Input: part model. Units: mm. Frame: model coordinates. Face numbers are marked on the shaded views. Coordinates: 2 decimals unless noted, no trailing zeros. Write each loop counter-clockwise with the first axis right and the second up, starting at its lowest first coordinate (ties: lowest second). Pieces come first, ordered by that corner, then holes.
1) Pin query (flat end, axial travel): pin 1 Ø1.5 at (x, y) = (4, 12.5) entering from +Z; pin 2 Ø1.6 at (x, y) = (6, 21) entering from -Z (3 decimals); pin 3 Ø0.8 at (x, z) = (-7, 1) entering from +Y; pin 4 Ø0.8 at (y, z) = (9, 0.5) entering from -X. Return the tip coordinate at first contact, or that it passes through.
2) Draft query along X for the marked faces 1, 2 and 3. Return one class per face: pulls with the +X half, pulls with the -X half, needs draft (parallel to the pull), parting line crosses it, or undercut.
3) Section query C-C (y = 16). Output: boundary loops of the cut face in (x, z).
4) Section query A-A (z = 1.9). Output: boundary loops of the cut face in (x, y).
5) Section query B-B (x = 2). Output: boundary loops of the cut face in (y, z).
6) Line query: L1, parallel to Y at x = -6, z = 1.1; L2, parallel to Z at x = -6.5, y = 4.75; L3, parallel to Y at x = 6, z = 2.15. Output: solid intervals per line, ascending.
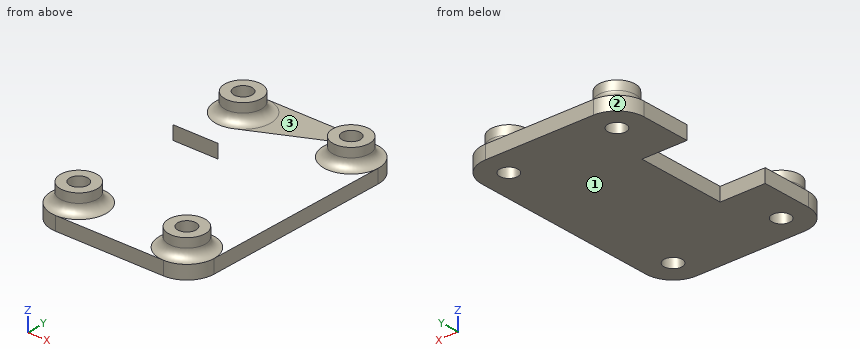
Autodesk Inventor part; units mm, degrees
ref_plane "YZ Plane" through (0, 0, 0) normal (1, 0, 0) x (0, 1, 0)
ref_plane "XZ Plane" through (0, 0, 0) normal (0, 1, 0) x (-1, 0, 0)
ref_plane "XY Plane" through (0, 0, 0) normal (0, 0, 1) x (1, 0, 0)
sketch "Náčrt1" plane through (0, 0, 0) normal (0, 0, 1) x (1, 0, 0)
  circle A0 centre (-6, 0) radius 1
  circle A1 centre (-6, 21) radius 1
  circle A2 centre (6, 0) radius 1
  circle A3 centre (6, 21) radius 1
  arc A4 (-6, 24) -> (-9, 21) centre (-6, 21) ccw
  arc A5 (9, 21) -> (6, 24) centre (6, 21) ccw
  arc A6 (6, -3) -> (9, 0) centre (6, 0) ccw
  arc A7 (-9, 0) -> (-6, -3) centre (-6, 0) ccw
  line L0 (-6, 24) -> (6, 24)
  line L1 (9, 21) -> (9, 0)
  line L2 (-6, -3) -> (6, -3)
  line L3 (-9, 15.5) -> (-4, 15.5)
  line L4 (-9, 5.5) -> (-4, 5.5)
  line L5 (-4, 15.5) -> (-4, 5.5)
  line L6 (-9, 21) -> (-9, 15.5)
  line L7 (-9, 5.5) -> (-9, 0)
  point P0 (0, 0)
  dimension "d0" = 2
  dimension "d2" = 2
  dimension "d4" = 19
  dimension "d5" = 2
  dimension "d6" = 2
  dimension "d7" = 2
  dimension "d8" = 2
  dimension "d9" = 4.5
  dimension "d10" = 5
extrude "Vysunutí1" add sketch "Náčrt1" along normal blind 1.5
sketch "Náčrt3" plane through (0, 0, 1.5) normal (0, 0, 1) x (1, 0, 0)
  circle A0 centre (-6, 21) radius 1
  circle A1 centre (-6, 21) radius 1
  circle A2 centre (6, 21) radius 1
  circle A3 centre (6, 21) radius 1
  circle A4 centre (6, 0) radius 1
  circle A5 centre (6, 0) radius 1
  circle A6 centre (-6, 0) radius 1
  circle A7 centre (-6, 21) radius 2
  circle A8 centre (6, 21) radius 2
  circle A9 centre (6, 0) radius 2
  circle A10 centre (-6, 0) radius 2
  point P0 (0, 0)
  dimension "d13" = 1
  dimension "d14" = 1
  dimension "d15" = 1
  dimension "d16" = 1
extrude "Vysunutí2" add sketch "Náčrt3" along normal blind 2
fillet "Zaoblení1" radius 1 4 edges at (-8, 21, 1.5) (4, 21, 1.5) (-8, 0, 1.5) (4, 0, 1.5)
properties part number "drzak_kamery2"
Answer:
1. pin 1: stops at z = 1.5
1. pin 2: passes through
1. pin 3: stops at y = 23.94
1. pin 4: stops at x = -4
2. face 1: needs draft
2. face 2: pulls with the -X half
2. face 3: undercut
3. outline: (-9, 0) - (9, 0) - (9, 1.5) - (-9, 1.5) - close
4. outline: circle Ø4.4 at (-6, 0); circle Ø4.4 at (-6, 21); circle Ø4.4 at (6, 0); circle Ø4.4 at (6, 21); hole circle Ø2 at (-6, 0); hole circle Ø2 at (-6, 21); hole circle Ø2 at (6, 0); hole circle Ø2 at (6, 21)
5. outline: (-3, 0) - (24, 0) - (24, 1.5) - (-3, 1.5) - close
6. L1: y = -3 to -1, 1 to 5.5, 15.5 to 20, 22 to 24
6. L2: z = 0 to 1.5
6. L3: y = -2.06 to -1, 1 to 2.06, 18.94 to 20, 22 to 23.06
